from build123d import *

# Parameters (mm, degrees)
SKETCH_1_R               = 9
SKETCH_1_R_2             = 6
EXTRUDE_1_DEPTH          = 3
CHAMFER_1_SIZE           = 0.5
SKETCH_2_W               = 2
SKETCH_2_H               = 2
CUT_EXTRUDE_1_DEPTH      = 14.076696831
PATTERN_CIRCULAR_1_COUNT = 4


with BuildPart() as part:
    # Эскиз1 → Бобышка-Вытянуть1 (new body)
    with BuildSketch(Plane.XY):
        Circle(SKETCH_1_R)
        Circle(SKETCH_1_R_2, mode=Mode.SUBTRACT)
    extrude(amount=EXTRUDE_1_DEPTH)

    # Фаска1
    chamfer_1_edges = [part.edges().sort_by_distance(p)[0] for p in [
        (-9, 0, 0),
        (-9, 0, 3),
        (-6, 0, 0),
        (-6, 0, 3),
    ]]
    chamfer(chamfer_1_edges, length=CHAMFER_1_SIZE)

    # Эскиз2 → Вырез-Вытянуть1 (cut, through all)
    with BuildSketch(Plane.XY.offset(3)):
        with Locations((0, 9)):
            Rectangle(SKETCH_2_W, SKETCH_2_H)
    cut_extrude_1 = extrude(amount=-CUT_EXTRUDE_1_DEPTH, mode=Mode.SUBTRACT)

    # Круговой массив1: Вырез-Вытянуть1 ×4 about axis
    pattern_circular_1_axis = Axis((0, 0, 0), (0, 0, 1))
    for i in range(1, PATTERN_CIRCULAR_1_COUNT):
        add(cut_extrude_1.rotate(pattern_circular_1_axis, i * 360 / PATTERN_CIRCULAR_1_COUNT), mode=Mode.SUBTRACT)


solid = part.part
Could you check a few things on this model? Use its own coordinates, in mm. A direction names the side the tool comes from. Give positions to 0.01 mm unless a question says otherwise; leave off trailing zeros. Order: outer loops, then holes, each group sorted by start corner. A loop starts at its lowest first (then second) coordinate and runs counter-clockwise, first axis right, second up. Notation, with made-up numbers: (35, 25) -> (83, 25) arc R27 ccw to (83, 41) -> close; hole circle Ø4 at (45, -12). An arc over 180 degrees is marked (long way). Answer in a Markdown table with one row per item. Add a question column.
Item 1: Imagine slicing it at C-C (z = 1.8). List the corners of the cut face in (x, y) for me, and give its area (3 significant figures).
Item 2: Please list where these lines run through material, in increasing order: probe 1 along Y at (x, z) = (0, 2.05); probe 2 along X at (y, z) = (4.25, 1.1); probe 3 along X at (y, z) = (5, 2.4).
Item 3: We'd pull the mould along Y, two halves only. Please class faces 6 (the flat face through (4, -6, 3)), 7 (the conical face through (6.048, -6.163, 2.865)), 8 (the flat face through (-8.5, 1, 1.5)): pulls with the +Y half, pulls with the -Y half, needs draft (parallel to the pull), parting line crosses it, or undercut.
Item 4: I'm going to push flat-ended pins straight in: P1, Ø0.8, axis at y = -8.5, z = 2, coming from the -X side; P2, Ø1, axis at x = 8.5, z = 2, coming from the -Y side; P3, Ø5, axis at x = -7, y = 6, coming from the +Z side; P4, Ø0.5, axis at y = 8.5, z = 1.5, coming from the +X side. Where does each tip first touch, or does it pass through?
Item 5: For faces 1 (the cylindrical face through (-6.304, 6.424, 1.486)), 2 (the flat face through (-1, 8.5, 1.5)), 3 (the flat face through (0, -8, 2)), 4 (the conical face through (-6.163, -6.048, 0.135)), 5 (the flat face through (8.5, -1, 1.5)), which set-ups out of +Z, -Z, +X, -X, +Y, -Y let a thin tool reach every point of the face, with its end or its side?
Item 6: Imagine slicing it at A-A (x = 0). List the corners of the cut face in (y, z) for me.
Result:
| question | item | result |
|---|---|---|
| 1 | outline | (-8.94, -1) arc R9 ccw to (-1, -8.94) -> (-1, -8) -> (1, -8) -> (1, -8.94) arc R9 ccw to (8.94, -1) -> (8, -1) -> (8, 1) -> (8.94, 1) arc R9 ccw to (1, 8.94) -> (1, 8) -> (-1, 8) -> (-1, 8.94) arc R9 ccw to (-8.94, 1) -> (-8, 1) -> (-8, -1) -> close; hole circle Ø12 at (0, 0) |
| 1 | area | 134 mm2 |
| 2 | probe 1 | -8 to -6, 6 to 8 |
| 2 | probe 2 | -7.93 to -4.24, 4.24 to 7.93 |
| 2 | probe 3 | -7.48 to -3.32, 3.32 to 7.48 |
| 3 | face 6 | needs draft |
| 3 | face 7 | pulls with the -Y half |
| 3 | face 8 | undercut |
| 4 | P1 | x = -3.92 |
| 4 | P2 | y = -4.12 |
| 4 | P3 | z = 3 |
| 4 | P4 | x = 3.6 |
| 5 | face 1 | +Z, -Z, -X, +Y |
| 5 | face 2 | +Z, -Z, +Y |
| 5 | face 3 | +Z, -Z, -Y |
| 5 | face 4 | -Z, -X, -Y |
| 5 | face 5 | +Z, -Z, +X |
| 6 | outline | (-8, 0) -> (-6.5, 0) -> (-6, 0.5) -> (-6, 2.5) -> (-6.5, 3) -> (-8, 3) -> close; (6, 0.5) -> (6.5, 0) -> (8, 0) -> (8, 3) -> (6.5, 3) -> (6, 2.5) -> close |
